Geometry check sheet. Reference: drawing and pictorial views, mm from the part's lowest x, y, z. Coordinates: 2 decimals unless noted, no trailing zeros. Loops run counter-clockwise (first coordinate to the right, second up) from the corner with the lowest first, then second, coordinate; pieces in that order, holes last. Notation, with made-up numbers: (1, 87) -> (7, 87) arc R12 cw to (7, 98) -> close; hole circle Ø11 at (76.25, 69). An arc over 180 degrees is marked (long way). Use CSV: the item, a comma, the result in double quotes.
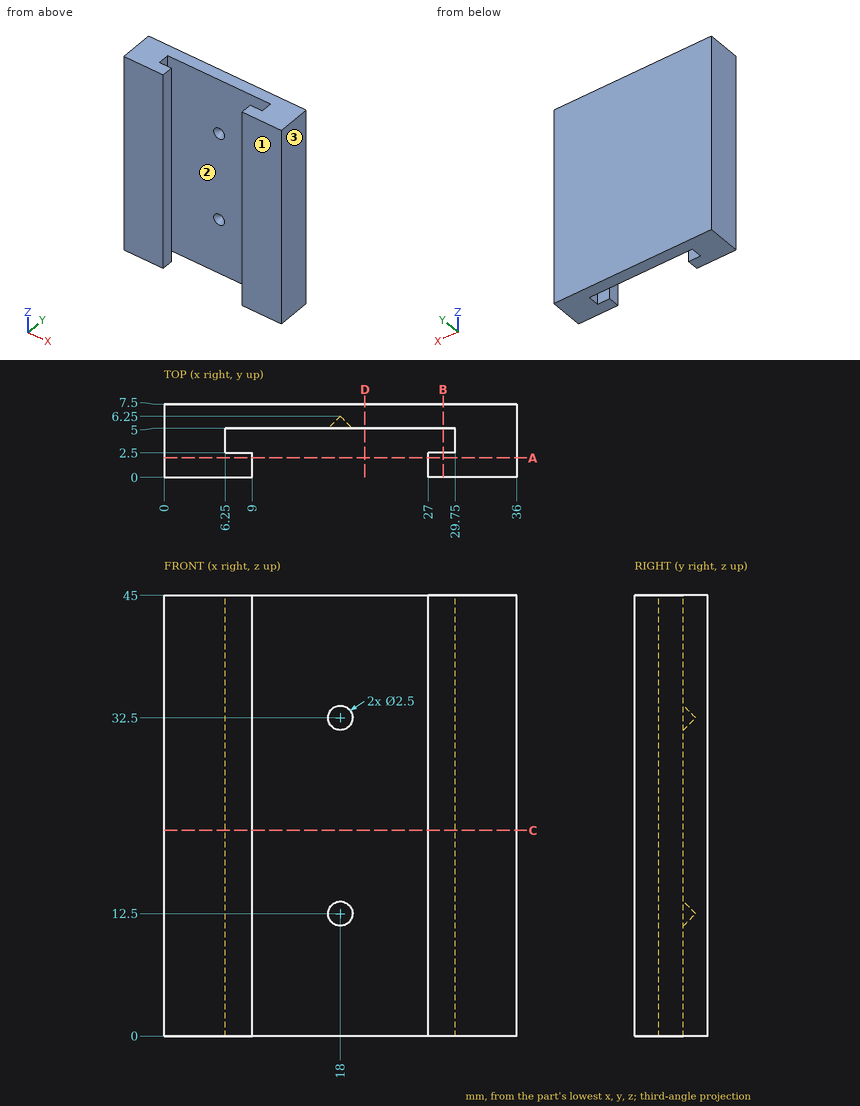
1) Thickness scan on line 1 along X through (y, z) = (2.75, 10.5); line 2 along Y through (x, z) = (6.5, 42); line 3 along Y through (x, z) = (25.5, 11.5). Record the ranges inside material, lowest first. Write a range as from..to.
Answer below:
line 1,"x = 0..6.25, 29.75..36"
line 2,"y = 0..2.5, 5..7.5"
line 3,"y = 5..7.5"
2) Cross-section at C-C on z = 21. Record the boundary of the cut face in (x, y).
Answer below:
outline,"(0, 0) -> (9, 0) -> (9, 2.5) -> (6.25, 2.5) -> (6.25, 5) -> (29.75, 5) -> (29.75, 2.5) -> (27, 2.5) -> (27, 0) -> (36, 0) -> (36, 7.5) -> (0, 7.5) -> close"
3) Cross-section at D-D on x = 20.5. Record the boundary of the cut face in (y, z).
Answer below:
outline,"(5, 0) -> (7.5, 0) -> (7.5, 45) -> (5, 45) -> close"
4) Cross-section at B-B on x = 28.5. Record the boundary of the cut face in (y, z).
Answer below:
outline,"(0, 0) -> (2.5, 0) -> (2.5, 45) -> (0, 45) -> close; (5, 0) -> (7.5, 0) -> (7.5, 45) -> (5, 45) -> close"
5) Cross-section at A-A on y = 2. Record the boundary of the cut face in (x, z), and give its area (3 significant figures).
Answer below:
outline,"(0, 0) -> (9, 0) -> (9, 45) -> (0, 45) -> close; (27, 0) -> (36, 0) -> (36, 45) -> (27, 45) -> close"
area,"810 mm²"
6) Draft check along Y on the marked faces 1, 2 and 3. Enter one of: released by +Y, released by -Y, zero draft, split by the parting line, or undercut.
Answer below:
face 1,"released by -Y"
face 2,"undercut"
face 3,"zero draft"
7) Go/stop test with flat-tipped pins: pin 1 Ø1.5 at (y, z) = (6.5, 39) entering from -X; pin 2 Ø2 at (x, z) = (22, 18.5) entering from -Y. Record where each tip stops, or that it passes through.
Answer below:
pin 1,"stops at x = 0"
pin 2,"stops at y = 5"
